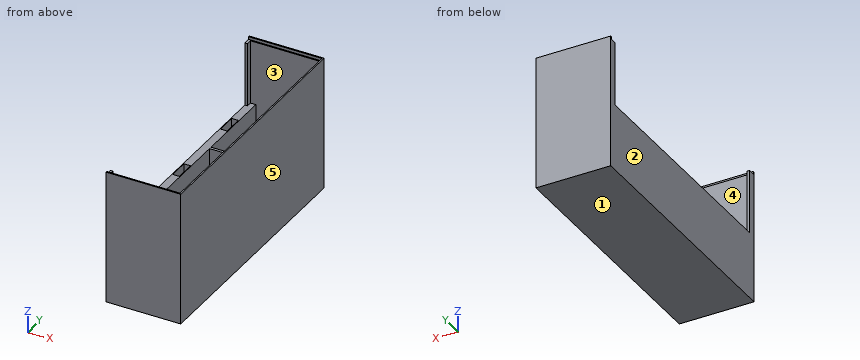
```python
from build123d import *

# Parameters (mm, degrees)
F0_W      = 260
F0_H      = 960
F1_DEPTH  = 250
F2_T      = -10
F3_W      = 240
F3_H      = 10
F4_DEPTH  = 240
F5_W      = 10
F5_H      = 20
F5_H_2    = 10
F5_H_3    = 920
F6_DEPTH  = 250
F0_W_2    = 20
F7_DEPTH  = 250
F8_W      = 25
F8_H      = 75
F9_DEPTH  = 75
F10_W     = 25
F10_H     = 10
F10_W_2   = 900
F11_DEPTH = 275


with BuildPart() as f1:
    # F0 (on Top) → F1 (new body)
    with BuildSketch(Plane.XY):
        Rectangle(F0_W, F0_H)
    extrude(amount=F1_DEPTH)

    # F2
    f2_openings = [f1.faces().sort_by_distance(p)[0] for p in [
        (0, 0, 250),
    ]]
    offset(amount=F2_T, openings=f2_openings)

    # F3 (on face) → F4 (join)
    with BuildSketch(Plane.XY.offset(10)):
        with Locations((0, -165)):
            Rectangle(F3_W, F3_H)
        with Locations((0, 165)):
            Rectangle(F3_W, F3_H)
    extrude(amount=F4_DEPTH)

    # F5 (on face) → F6 (join)
    with BuildSketch(Plane.XY.offset(250)):
        with Locations((-145, -460)):
            Rectangle(F5_W, F5_H)
        Polygon((-150, -480), (120, -480), (120, -470), (-120, -470), (-140, -470), (-150, -470), align=None)
        with Locations((125, -475)):
            Rectangle(F5_W, F5_H_2)
        with Locations((125, -465)):
            Rectangle(F5_W, F5_H_2)
        with Locations((125, 0)):
            Rectangle(F5_W, F5_H_3)
        with Locations((125, 465)):
            Rectangle(F5_W, F5_H_2)
        with Locations((125, 475)):
            Rectangle(F5_W, F5_H_2)
        Polygon((-120, 470), (120, 470), (120, 480), (-150, 480), (-150, 470), (-140, 470), align=None)
        with Locations((-145, 460)):
            Rectangle(F5_W, F5_H)
    extrude(amount=F6_DEPTH)

    # F0 (on Top) → F7 (join)
    with BuildSketch(Plane.XY):
        with Locations((-140, 0)):
            Rectangle(F0_W_2, F0_H)
    extrude(amount=F7_DEPTH)

    # F8 (on face) → F9 (cut)
    with BuildSketch(Plane.XY.offset(250)):
        with Locations((-135, 320)):
            Rectangle(F8_W, F8_H)
        with Locations((-135, 0)):
            Rectangle(F8_W, F8_H)
        with Locations((-135, -320)):
            Rectangle(F8_W, F8_H)
    extrude(amount=-F9_DEPTH, mode=Mode.SUBTRACT)

    # F10 (on face) → F11 (cut)
    with BuildSketch(Plane(origin=(-150, 0, 0), x_dir=(0, -1, 0), z_dir=(-1, 0, 0))):
        with Locations((462.5, 495)):
            Rectangle(F10_W, F10_H)
        with Locations((-462.5, 495)):
            Rectangle(F10_W, F10_H)
        with Locations((0, 495)):
            Rectangle(F10_W_2, F10_H)
    extrude(amount=-F11_DEPTH, mode=Mode.SUBTRACT)


solid = f1.part
```
Can you work these out from the model? Positions are in its coordinate system, mm. Face numbers are marked on the shaded views. A direction names the side the tool comes from. Round coordinates to 2 decimals unless told otherwise and drop trailing zeros. Order: outer loops, then holes, each group sorted by start corner. A loop starts at its lowest first (then second) coordinate and runs counter-clockwise, first axis right, second up. Notation, with made-up numbers: (-2, 42) -> (24, 42) arc R10 ccw to (24, 50) -> close; hole circle Ø1 at (15.25, 69). An arc over 180 degrees is marked (long way). Return JSON: item names as keys, results as strings. Group by question number.
1. If we section it at D-D, the plane y = -390.5: Write out the boundary of the cut face in (x, z).
2. If we section it at A-A, the plane y = -292.5: Write out the boundary of the cut face in (x, z), then the cut area to 3 significant figures.
3. If we section it at B-B, the plane z = 284: Write out the boundary of the cut face in (x, y).
4. Which directions (+Z, -Z, +X, -X, +Y, -Y) give clear straight access to the entire face, cutting with the end or side of a thin tool? Please do the marked faces 4 and 5.
5. Will these pins go through, and if not, where does the flat tip stop? pin 1 (4 mm diameter, centred on x = -34.5, y = -357.5, fed in from +Z); pin 2 (10 mm diameter, centred on y = 177, z = 363.5, fed in from -X); pin 3 (7.5 mm diameter, centred on x = -138.5, y = -321, fed in from +Z).
6. If we section it at C-C, the plane x = 63.5: Write out the boundary of the cut face in (y, z), then the cut area to 3 significant figures.
7. We'd pull the mould along X, two halves only. Please class the marked faces 1, 2 and 3: released by +X, released by -X, zero draft, split by the parting line, or undercut.
8. I need wall thicknesses on line 1 (Y direction, x = 116, z = 69); line 2 (X direction, y = -294.5, z = 222); line 3 (Y direction, x = -25, z = 431). Which ranges of each line are inside material? Lowest first, please. Write a range as [from, to].
Output values:
{
 "1": {"outline": "(-150, 0) -> (130, 0) -> (130, 500) -> (125, 500) -> (125, 490) -> (120, 490) -> (120, 10) -> (-120, 10) -> (-120, 250) -> (-150, 250) -> close"},
 "2": {"outline": "(-150, 0) -> (130, 0) -> (130, 500) -> (125, 500) -> (125, 490) -> (120, 490) -> (120, 10) -> (-120, 10) -> (-120, 250) -> (-122.5, 250) -> (-122.5, 175) -> (-147.5, 175) -> (-147.5, 250) -> (-150, 250) -> close", "area": "13,000 mm²"},
 "3": {"outline": "(-150, -480) -> (130, -480) -> (130, 480) -> (-150, 480) -> (-150, 450) -> (-140, 450) -> (-140, 470) -> (120, 470) -> (120, -470) -> (-140, -470) -> (-140, -450) -> (-150, -450) -> close"},
 "4": {"face 4": "+Z", "face 5": "+Z, -Z, +X, +Y, -Y"},
 "5": {"pin 1": "z = 10", "pin 2": "x = 120", "pin 3": "z = 175"},
 "6": {"outline": "(-480, 0) -> (480, 0) -> (480, 500) -> (475, 500) -> (475, 490) -> (470, 490) -> (470, 10) -> (170, 10) -> (170, 250) -> (160, 250) -> (160, 10) -> (-160, 10) -> (-160, 250) -> (-170, 250) -> (-170, 10) -> (-470, 10) -> (-470, 490) -> (-475, 490) -> (-475, 500) -> (-480, 500) -> close", "area": "24,100 mm²"},
 "7": {"face 1": "zero draft", "face 2": "released by -X", "face 3": "undercut"},
 "8": {"line 1": "[-480, -470], [-170, -160], [160, 170], [470, 480]", "line 2": "[-150, -147.5], [-122.5, -120], [120, 130]", "line 3": "[-480, -470], [470, 480]"}
}
